```python
from build123d import *

# Parameters (mm, degrees)
SKETCH_1_W          = 20
SKETCH_1_H          = 7
SKETCH_1_R          = 1.65
EXTRUDE_1_DEPTH     = 12
SKETCH_2_W          = 8.5
SKETCH_2_H          = 5.3
CUT_EXTRUDE_1_DEPTH = 12
SKETCH_3_W          = 9
SKETCH_3_H          = 3.5
CUT_EXTRUDE_2_DEPTH = 12
FILLET_1_R          = 3
FILLET_2_R          = 3
FILLET_3_R          = 1
SKETCH_5_R          = 1.65
SKETCH_5_R_2        = 1.5
EXTRUDE_2_DEPTH     = 3.35


with BuildPart() as part:
    # 草图1 → 凸台-拉伸1 (new body)
    with BuildSketch(Plane.XY):
        Rectangle(SKETCH_1_W, SKETCH_1_H)
        with Locations((-6.5, 0)):
            Circle(SKETCH_1_R, mode=Mode.SUBTRACT)
        with Locations(Location((6.5, 0, 0), (0, 0, 180))):
            Circle(SKETCH_1_R, mode=Mode.SUBTRACT)
    extrude(amount=EXTRUDE_1_DEPTH)

    # 草图2 → 切除-拉伸1 (cut)
    with BuildSketch(Plane(origin=(0, 3.5, 0), x_dir=(1, 0, 0), z_dir=(0, 1, 0))):
        with Locations((-5.75, -6)):
            Rectangle(SKETCH_2_W, SKETCH_2_H)
    extrude(amount=-CUT_EXTRUDE_1_DEPTH, mode=Mode.SUBTRACT)

    # 草图3 → 切除-拉伸2 (cut)
    with BuildSketch(Plane(origin=(0, 3.5, 0), x_dir=(1, 0, 0), z_dir=(0, 1, 0))):
        with Locations((5.5, -1.75)):
            Rectangle(SKETCH_3_W, SKETCH_3_H)
        with Locations((5.5, -10.25)):
            Rectangle(SKETCH_3_W, SKETCH_3_H)
    extrude(amount=-CUT_EXTRUDE_2_DEPTH, mode=Mode.SUBTRACT)

    # 圆角1
    fillet_1_edges = [part.edges().sort_by_distance(p)[0] for p in [
        (-10, -3.5, 1.675),
        (-10, 3.5, 1.675),
        (10, -3.5, 6),
        (10, 3.5, 6),
        (-10, -3.5, 10.325),
        (-10, 3.5, 10.325),
    ]]
    fillet(fillet_1_edges, radius=FILLET_1_R)

    # 圆角2
    fillet_2_edges = [part.edges().sort_by_distance(p)[0] for p in [
        (1, 0, 0),
        (1, 0, 12),
    ]]
    fillet(fillet_2_edges, radius=FILLET_2_R)

    # 圆角3
    fillet_3_edges = [part.edges().sort_by_distance(p)[0] for p in [
        (1, 0, 3.5),
        (1, 0, 8.5),
    ]]
    fillet(fillet_3_edges, radius=FILLET_3_R)

    # 草图5 → 凸台-拉伸2 (add)
    with BuildSketch(Plane(origin=(0, 0, 8.65), x_dir=(-1, 0, 0), z_dir=(0, 0, -1))):
        with Locations((6.5, 0)):
            Circle(SKETCH_5_R)
        with Locations((6.5, 0)):
            Circle(SKETCH_5_R_2, mode=Mode.SUBTRACT)
    extrude(amount=-EXTRUDE_2_DEPTH)


solid = part.part
```
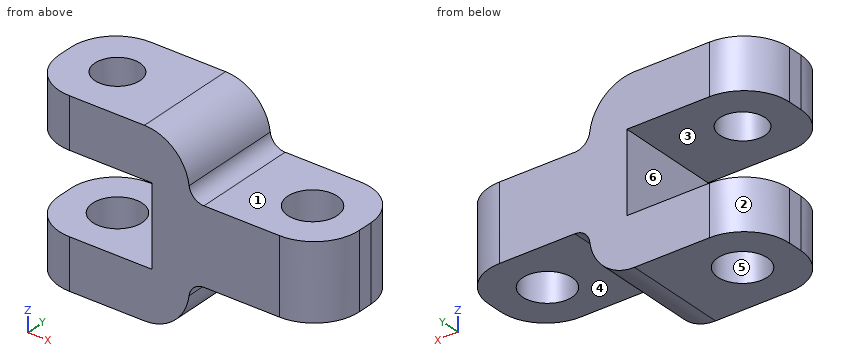
Read the model definition and answer for the solid it produces. Units are mm, in the model's axes. Face numbers are marked on the shaded views. A direction names the side the tool comes from. Coordinates: 2 decimals unless noted, no trailing zeros. Order: outer loops, then holes, each group sorted by start corner. A loop starts at its lowest first (then second) coordinate and runs counter-clockwise, first axis right, second up. Notation, with made-up numbers: (29.5, 9) - (77.5, 9) arc R19 cw to (77.5, 22) - close; hole circle Ø6 at (69, 7.5). An arc over 180 degrees is marked (long way). Answer as a JSON object with one key per item and string values. Group by question number.
Item 1: Section A-A (z = 5) is taken. Give the vertices of the cut face in (x, y), plus the area to 3 significant figures.
Item 2: Section D-D (y = 0) is taken. State how many separate pieces and enclosed holes the cut face has, plus the area to 3 significant figures.
Item 3: Section C-C (x = -6.5) is taken. Give the vertices of the cut face in (y, z).
Item 4: The mould has two halves that part along Z. Classify the marked faces 1, 2 and 3: +Z half, -Z half, draft (parallel to the pull), parting line (faces both ways), or undercut.
Item 5: Flat-ended cylindrical pins translate along their axes: P1, Ø2.5, axis at y = 1, z = 5.5, coming from the -X side; P2, Ø3.5, axis at x = 5.5, y = -1, coming from the +Z side; P3, Ø3, axis at y = 2, z = 4.5, coming from the -X side. Find the tip coordinate at first contact, or state that the pin passes through.
Item 6: Consider probe 1 along Z at (x, y) = (-3.75, 0); probe 2 along Y at (x, z) = (6.5, 6.7); probe 3 along Y at (x, z) = (-6.5, 10.55). Determine where each line is inside the solid, lowest interval first. Write a range as from..to.
Item 7: Section B-B (x = 6.5) is taken. Give the vertices of the cut face in (y, z).
Item 8: A tool of negligible diameter and unlimited length cuts with its end or side. For the marked faces 4, 5 and 6, from which of +Z, -Z, +X, -X, +Y, -Y can it reach the whole face along a straight path? Write none if from no direction.
Results are:
{
 "1": {"outline": "(-1.5, -3.5) - (7, -3.5) arc R3 ccw to (10, -0.5) - (10, 0.5) arc R3 ccw to (7, 3.5) - (-1.5, 3.5) - close; hole circle Ø3.3 at (6.5, 0)", "area": "68.1 mm^2"},
 "2": {"separate pieces": "4", "enclosed holes": "0", "area": "90.9 mm^2"},
 "3": {"outline": "(-3.5, 0) - (-1.65, 0) - (-1.65, 3.35) - (-3.5, 3.35) - close; (-3.5, 8.65) - (-1.5, 8.65) - (-1.5, 12) - (-3.5, 12) - close; (1.5, 8.65) - (3.5, 8.65) - (3.5, 12) - (1.5, 12) - close; (1.65, 0) - (3.5, 0) - (3.5, 3.35) - (1.65, 3.35) - close"},
 "4": {"face 1": "+Z half", "face 2": "draft", "face 3": "undercut"},
 "5": {"P1": "stops at x = -1.5", "P2": "stops at z = 8.5", "P3": "stops at x = -9.95"},
 "6": {"probe 1": "z = 0..3.35, 8.65..12", "probe 2": "y = -3.5..-1.65, 1.65..3.5", "probe 3": "y = -3.5..-1.5, 1.5..3.5"},
 "7": {"outline": "(-3.5, 3.5) - (-1.65, 3.5) - (-1.65, 8.5) - (-3.5, 8.5) - close; (1.65, 3.5) - (3.5, 3.5) - (3.5, 8.5) - (1.65, 8.5) - close"},
 "8": {"face 4": "-Z, +X, +Y, -Y", "face 5": "-Z", "face 6": "-X, +Y, -Y"}
}
